Work out the finished part from the listing and answer in its coordinate system (mm). A direction names the side the tool comes from. Round coordinates to 2 decimals unless told otherwise and drop trailing zeros. Order: outer loops, then holes, each group sorted by start corner. A loop starts at its lowest first (then second) coordinate and runs counter-clockwise, first axis right, second up. Notation, with made-up numbers: (-16, 81) - (26, 81) arc R6 ccw to (26, 85) - close; hole circle Ø5 at (13.5, 46.5). An arc over 180 degrees is marked (long way). Put each result on its own line as item: value.
```python
from build123d import *

# Parameters (mm, degrees)
F0_R     = 31.618646
F1_DEPTH = 100
F2_R     = 15
F3_DEPTH = 25
F4_R     = 4.5
F5_DEPTH = 50
F6_R     = 15
F7_DEPTH = 25
F8_R     = 4.5
F9_DEPTH = 50


with BuildPart() as f1:
    # F0 (on Top) → F1 (new body)
    with BuildSketch(Plane.XY):
        Circle(F0_R)
    extrude(amount=F1_DEPTH)

    # F2 (on face) → F3 (join)
    with BuildSketch(Plane(origin=(0, 0, 0), x_dir=(1, 0, 0), z_dir=(0, 0, -1))):
        Circle(F2_R)
    extrude(amount=F3_DEPTH)

    # F4 (on face) → F5 (join)
    with BuildSketch(Plane(origin=(0, 0, -25), x_dir=(1, 0, 0), z_dir=(0, 0, -1))):
        Circle(F4_R)
    extrude(amount=F5_DEPTH)

    # F6 (on face) → F7 (join)
    with BuildSketch(Plane.XY.offset(100)):
        Circle(F6_R)
    extrude(amount=F7_DEPTH)

    # F8 (on face) → F9 (join)
    with BuildSketch(Plane.XY.offset(125)):
        Circle(F8_R)
    extrude(amount=F9_DEPTH)


solid = f1.part
```
1) For faces 1 (the cylindrical face through (30.159, 9.497, 49.3)), 2 (the flat face through (3, -4, -25)), 3 (the flat face through (3, 4, 125)), determine the directions among +Z, -Z, +X, -X, +Y, -Y from which every point of the face is accessible in a straight line to the end or side of a thin tool.
Findings below:
face 1: +Z, -Z
face 2: -Z
face 3: +Z
2) Given pin 1 Ø2 at (x, y) = (15.5, -18.5) entering from -Z; pin 2 Ø1.5 at (x, y) = (-6, -4) entering from +Z; pin 3 Ø3 at (x, z) = (0.5, 13) entering from -Y, each flat-ended and moving along its own axis, determine where each tip first touches the part or whether it passes through.
Findings below:
pin 1: stops at z = 0
pin 2: stops at z = 125
pin 3: stops at y = -31.62
3) A cutting plane is placed at D-D on z = 64.5. Write down the section's boundary in (x, y), then the cut area to 3 significant figures.
Findings below:
outline: circle Ø63.24 at (0, 0)
area: 3,140 mm2
4) A cutting plane is placed at C-C on z = 119. Write down the section's boundary in (x, y), then the cut area to 3 significant figures.
Findings below:
outline: circle Ø30 at (0, 0)
area: 707 mm2
5) A cutting plane is placed at A-A on x = 0. Write down the section's boundary in (y, z), then the cut area to 3 significant figures.
Findings below:
outline: (-31.62, 0) - (-15, 0) - (-15, -25) - (-4.5, -25) - (-4.5, -75) - (4.5, -75) - (4.5, -25) - (15, -25) - (15, 0) - (31.62, 0) - (31.62, 100) - (15, 100) - (15, 125) - (4.5, 125) - (4.5, 175) - (-4.5, 175) - (-4.5, 125) - (-15, 125) - (-15, 100) - (-31.62, 100) - close
area: 8,720 mm2
6) Straight lines are drawn through the part: L1, parallel to Z at x = 19.5, y = 19; L2, parallel to Y at x = -1, z = 93; L3, parallel to Z at x = -8, y = -5. For each, find the intervals that lie inside material, in ascending order. Write a range as from..to.
Findings below:
L1: z = 0..100
L2: y = -31.6..31.6
L3: z = -25..125
